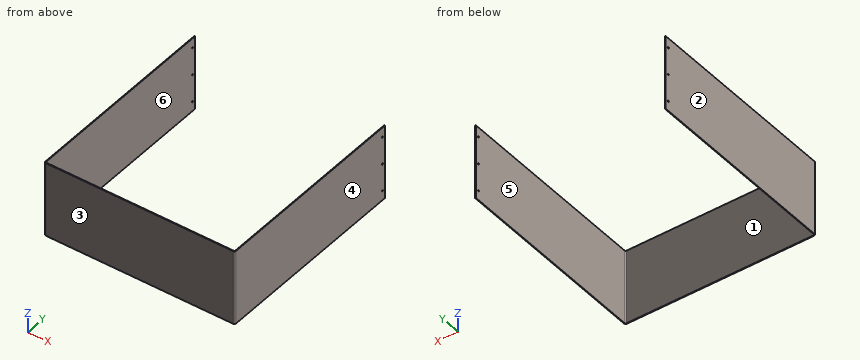
from build123d import *

# Parameters (mm, degrees)
SZKIC1_W                             = 546
SZKIC1_H                             = 216
ODGI_CIE_BAZOWE1_DEPTH               = 2
ODGI_CIE_KRAW_DZI1_STRIP_W           = 14
ODGI_CIE_KRAW_DZI1_STRIP_H           = 2
ODGI_CIE_KRAW_DZI1_STRIP_CUT_DEPTH   = 216
ODGI_CIE_KRAW_DZI1_STRIP_2_W         = 14
ODGI_CIE_KRAW_DZI1_STRIP_2_H         = 2
ODGI_CIE_KRAW_DZI1_STRIP_CUT_2_DEPTH = 216
ODGI_CIE_KRAW_DZI1_DEPTH             = 216
ODGI_CIE_KRAW_DZI1_BEND_DEPTH        = 216
SZKIC12_R                            = 2.1
WYTNIJ_WYCI_GNI_CIE1_DEPTH           = 806.138497403


# Sheet-metal steps are written as plain solids
with BuildPart() as part:
    # Szkic1 → Odgięcie bazowe1 (new body)
    with BuildSketch(Plane(origin=(0, 0, 0), x_dir=(1, 0, 0), z_dir=(0, 1, 0))):
        Rectangle(SZKIC1_W, SZKIC1_H)
    extrude(amount=-ODGI_CIE_BAZOWE1_DEPTH)

    # Odgięcie krawędzi1 strip (across the edge) → Odgięcie krawędzi1 strip cut (cut)
    with BuildSketch(Plane(origin=(-273, 0, -108), x_dir=(1, 0, 0), z_dir=(0, 0, 1))):
        with Locations((-4, -1)):
            Rectangle(ODGI_CIE_KRAW_DZI1_STRIP_W, ODGI_CIE_KRAW_DZI1_STRIP_H)
    extrude(amount=ODGI_CIE_KRAW_DZI1_STRIP_CUT_DEPTH, mode=Mode.SUBTRACT)

    # Odgięcie krawędzi1 strip 2 (across the edge) → Odgięcie krawędzi1 strip cut 2 (cut)
    with BuildSketch(Plane(origin=(273, 0, 108), x_dir=(-1, 0, 0), z_dir=(0, 0, -1))):
        with Locations((-4, -1)):
            Rectangle(ODGI_CIE_KRAW_DZI1_STRIP_2_W, ODGI_CIE_KRAW_DZI1_STRIP_2_H)
    extrude(amount=ODGI_CIE_KRAW_DZI1_STRIP_CUT_2_DEPTH, mode=Mode.SUBTRACT)

    # Odgięcie krawędzi1 section (across the edge) → Odgięcie krawędzi1 (add)
    with BuildSketch(Plane(origin=(-273, 0, -108), x_dir=(1, 0, 0), z_dir=(0, 0, 1))):
        with BuildLine():
            Line((-2, 3), (-2, 578))
            Line((-2, 578), (0, 578))
            Line((0, 578), (0, 3))
            ThreePointArc((0, 3), (0.878679656, 0.878679656), (3, 0))
            Line((3, 0), (3, -2))
            ThreePointArc((3, -2), (-0.535533906, -0.535533906), (-2, 3))
        make_face()
    extrude(amount=ODGI_CIE_KRAW_DZI1_DEPTH)

    # Odgięcie krawędzi1 section 2 (across the edge) → Odgięcie krawędzi1 bend (add)
    with BuildSketch(Plane(origin=(273, 0, 108), x_dir=(-1, 0, 0), z_dir=(0, 0, -1))):
        with BuildLine():
            Line((-2, 3), (-2, 578))
            Line((-2, 578), (0, 578))
            Line((0, 578), (0, 3))
            ThreePointArc((0, 3), (0.878679656, 0.878679656), (3, 0))
            Line((3, 0), (3, -2))
            ThreePointArc((3, -2), (-0.535533906, -0.535533906), (-2, 3))
        make_face()
    extrude(amount=ODGI_CIE_KRAW_DZI1_BEND_DEPTH)

    # Szkic12 → Wytnij-wyciągnięcie1 (cut, through all)
    with BuildSketch(Plane.ZY.offset(275)):
        with Locations(Location((0, 568, 0), (0, 0, 270))):
            Circle(SZKIC12_R)
        with Locations(Location((80, 568, 0), (0, 0, 270))):
            Circle(SZKIC12_R)
        with Locations(Location((-80, 568, 0), (0, 0, 270))):
            Circle(SZKIC12_R)
    extrude(amount=-WYTNIJ_WYCI_GNI_CIE1_DEPTH, mode=Mode.SUBTRACT)


solid = part.part
Here's how the part is built. I have some questions about the finished solid (model axes, mm). Face numbers are marked on the shaded views. A direction names the side the tool comes from. Coordinates: 2 decimals unless noted, no trailing zeros. Order: outer loops, then holes, each group sorted by start corner. A loop starts at its lowest first (then second) coordinate and runs counter-clockwise, first axis right, second up.
Item 1: If we section it at B-B on z = 54.5: List the corners of the cut face in (x, y) for me, plus the area to 3 significant figures.
Result sheet:
outline: (-275, 3) arc R5 ccw to (-270, -2) - (270, -2) arc R5 ccw to (275, 3) - (275, 578) - (273, 578) - (273, 3) arc R3 cw to (270, 0) - (-270, 0) arc R3 cw to (-273, 3) - (-273, 578) - (-275, 578) - close
area: 3,410 mm2
Item 2: If we mould it in two halves opening along X, with no side actions, what happens to the marked faces 3, 4, 5 and 6? For each: +X half, -X half, draft (parallel to the pull), parting line (faces both ways), or undercut.
Result sheet:
face 3: draft
face 4: +X half
face 5: undercut
face 6: undercut
Item 3: I need wall thicknesses on line 1 (Z direction, x = 274.6, y = 568); line 2 (X direction, y = 344, z = 56); line 3 (Y direction, x = -68, z = -46). Which ranges of each line are inside material? Lowest first, please.
Result sheet:
line 1: z = -108 to -82.1, -77.9 to -2.1, 2.1 to 77.9, 82.1 to 108
line 2: x = -275 to -273, 273 to 275
line 3: y = -2 to 0
Item 4: If we section it at C-C on x = -156: List the corners of the cut face in (y, z) for me, plus the area to 3 significant figures.
Result sheet:
outline: (-2, -108) - (0, -108) - (0, 108) - (-2, 108) - close
area: 432 mm2
Item 5: If we section it at A-A on y = 219: List the corners of the cut face in (x, z) for me, plus the area to 3 significant figures.
Result sheet:
outline: (-275, -108) - (-273, -108) - (-273, 108) - (-275, 108) - close; (273, -108) - (275, -108) - (275, 108) - (273, 108) - close
area: 864 mm2
Item 6: For P1, Ø6, axis at x = -117.5, z = -5, coming from the +Y side, with a flat end and sliding along its axis, tell me the tip position at first contact or that it passes through.
Result sheet:
P1: stops at y = 0
Item 7: For the marked faces 1 and 2, which set-ups out of +Z, -Z, +X, -X, +Y, -Y let a thin tool reach every point of the face, with its end or its side?
Result sheet:
face 1: +Z, -Z, +Y
face 2: +Z, -Z, -X, +Y, -Y
